from build123d import *

# Parameters (mm, degrees)
F0_W     = 101.6
F0_H     = 101.6
F1_DEPTH = 6.35
F2_W     = 50.8
F2_H     = 50.8
F3_DEPTH = 25.4
F4_R     = 19.05
F5_DEPTH = 31.751


with BuildPart() as f1:
    # F0 (on Front) → F1 (new body)
    with BuildSketch(Plane.XZ):
        with Locations((50.8, 50.8)):
            Rectangle(F0_W, F0_H)
    extrude(amount=F1_DEPTH)

    # F2 (on face) → F3 (join)
    with BuildSketch(Plane.XZ.offset(6.35)):
        with Locations((50.8, 50.8)):
            Rectangle(F2_W, F2_H)
    extrude(amount=F3_DEPTH)

    # F4 (on face) → F5 (cut, through all)
    with BuildSketch(Plane.XZ.offset(31.75)):
        with Locations((50.8, 50.8)):
            Circle(F4_R)
    extrude(amount=-F5_DEPTH, mode=Mode.SUBTRACT)


solid = f1.part
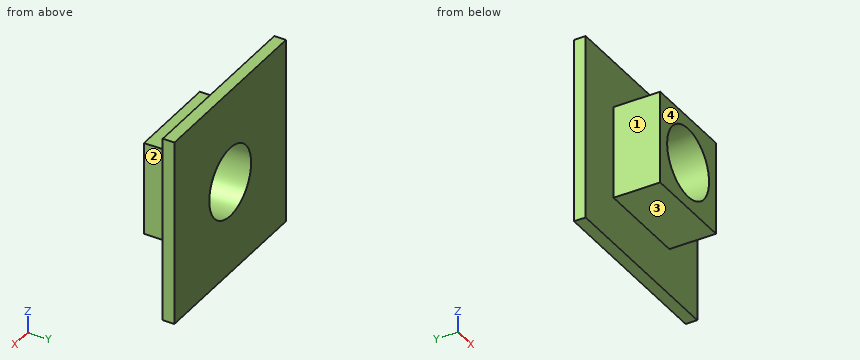
Design review of the part built by this model. Coordinates are the model's own, in mm. Face numbers are marked on the shaded views. A direction names the side the tool comes from. Round coordinates to 2 decimals unless told otherwise and drop trailing zeros. Write each loop counter-clockwise with the first axis right and the second up, starting at its lowest first coordinate (ties: lowest second). Pieces come first, ordered by that corner, then holes.
Item 1: For the marked faces 1, 2, 3 and 4, list the 3-axis set-ups (+Z, -Z, +X, -X, +Y, -Y) from which the entire face can be reached by the end or side of a thin tool; tool diameter is ignored.
Item 2: For pin 1 Ø10 at (x, y) = (66.5, -13) entering from +Z; pin 2 Ø8 at (x, z) = (82, 54.5) entering from +Y; pin 3 Ø7.5 at (y, z) = (-16.5, 54) entering from -X; pin 4 Ø5 at (y, z) = (-18.5, 26.5) entering from +X, all flat-tipped, find the tip position at first contact; note any pin that passes through.
Item 3: Wall thickness on L1, parallel to Z at x = 50, y = -15; L2, parallel to Y at x = 87, z = 54: over which ranges is each line inside the solid? List them lowest first.
Item 4: Consider section C-C on x = 50.8. Give the boundary of the cut face in (y, z), and give its area (3 significant figures).
Item 5: Consider section D-D on x = 27.5. Give the boundary of the cut face in (y, z).
Item 6: Consider section B-B on z = 50.8. Give the boundary of the cut face in (x, y).
Item 7: Consider section A-A on y = -17.5. Give the boundary of the cut face in (x, z), and give its area (3 significant figures).
Check values:
1. face 1: +Z, -Z, -X, -Y
1. face 2: +Z, -Z, +X, -Y
1. face 3: -Z, +X, -X, -Y
1. face 4: +Z, -Z, +X, -X, -Y
2. pin 1: stops at z = 76.2
2. pin 2: stops at y = 0
2. pin 3: stops at x = 25.4
2. pin 4: stops at x = 76.2
3. L1: z = 25.4 to 31.77, 69.83 to 76.2
3. L2: y = -6.35 to 0
4. outline: (-31.75, 25.4) - (-6.35, 25.4) - (-6.35, 0) - (0, 0) - (0, 31.75) - (-31.75, 31.75) - close; (-31.75, 69.85) - (0, 69.85) - (0, 101.6) - (-6.35, 101.6) - (-6.35, 76.2) - (-31.75, 76.2) - close
4. area: 726 mm2
5. outline: (-31.75, 25.4) - (-6.35, 25.4) - (-6.35, 0) - (0, 0) - (0, 101.6) - (-6.35, 101.6) - (-6.35, 76.2) - (-31.75, 76.2) - close
6. outline: (0, -6.35) - (25.4, -6.35) - (25.4, -31.75) - (31.75, -31.75) - (31.75, 0) - (0, 0) - close; (69.85, -31.75) - (76.2, -31.75) - (76.2, -6.35) - (101.6, -6.35) - (101.6, 0) - (69.85, 0) - close
7. outline: (25.4, 25.4) - (76.2, 25.4) - (76.2, 76.2) - (25.4, 76.2) - close; hole circle Ø38.1 at (50.8, 50.8)
7. area: 1,440 mm2
